Model file for the job. Use its own axes, mm. Face numbers are marked on the shaded views. Coordinates: 2 decimals unless noted, no trailing zeros. Write each loop counter-clockwise with the first axis right and the second up, starting at its lowest first coordinate (ties: lowest second). Pieces come first, ordered by that corner, then holes. Notation, with made-up numbers: M 19,-25.5 L 44,-25.5 A24 cw 44,-0.5 Z; hole C 41,-18.75 d5. An arc over 180 degrees is marked long. Use CSV: the item, a comma, the result in double quotes. Start each with the question number.
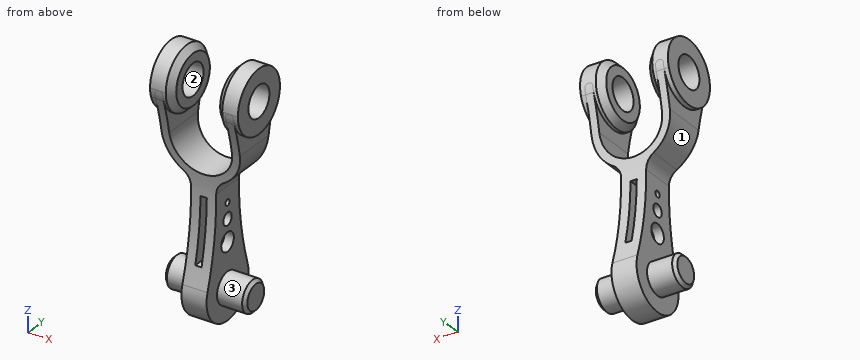
from build123d import *

# Parameters (mm, degrees)
F1_DEPTH  = 19.05
F3_R      = 12.7
F4_DEPTH  = 17.78
F2_R      = 6.35
F6_DEPTH  = 38.1
F5_W      = 17.78
F5_H      = 38.1
F7_DEPTH  = 19.05
F8_SIZE   = 2.54
F10_DEPTH = 5.08
F11_R     = 6.35
F12_DEPTH = 16.51
F13_SIZE  = 1.27
F15_DEPTH = 38.1
F16_W     = 2.54
F16_H     = 25.4
F17_DEPTH = 25.4
F18_R     = 3.81
F18_R_2   = 2.54
F18_R_3   = 1.27
F19_DEPTH = 12.7
F20_ANGLE = 179.9946913403


with BuildPart() as f1:
    # F0 (on Front) → F1 (new body, symmetric)
    with BuildSketch(Plane.XZ):
        with BuildLine():
            ThreePointArc((-5.08, -13.9496366999), (-5.9049678847, -17.0795760164), (-8.1655181496, -19.3962556739))
            ThreePointArc((-8.1655181496, -19.3962556739), (-13.8198807904, -25.1910159629), (-15.8833905736, -33.02))
            Line((-15.8833905736, -33.02), (-15.8833905736, -49.276))
            ThreePointArc((-15.8833905736, -49.276), (-15.4370213081, -50.3536307345), (-14.3593905736, -50.8))
            Line((-14.3593905736, -50.8), (-14.224, -50.8))
            ThreePointArc((-14.224, -50.8), (-13.1463692655, -50.3536307345), (-12.7, -49.276))
            Line((-12.7, -49.276), (-12.7, -33.02))
            ThreePointArc((-12.7, -33.02), (0, -20.32), (12.7, -33.02))
            Line((12.7, -33.02), (12.7, -49.276))
            ThreePointArc((12.7, -49.276), (13.1463692655, -50.3536307345), (14.224, -50.8))
            Line((14.224, -50.8), (14.3593905736, -50.8))
            ThreePointArc((14.3593905736, -50.8), (15.4370213081, -50.3536307345), (15.8833905736, -49.276))
            Line((15.8833905736, -49.276), (15.8833905736, -33.02))
            ThreePointArc((15.8833905736, -33.02), (13.8198807904, -25.1910159629), (8.1655181496, -19.3962556739))
            ThreePointArc((8.1655181496, -19.3962556739), (5.9049678847, -17.0795760164), (5.08, -13.9496366999))
            Line((5.08, -13.9496366999), (5.08, 2.3491094791))
            Line((5.08, 2.3491094791), (-5.08, 2.3491094791))
            Line((-5.08, 2.3491094791), (-5.08, -13.9496366999))
        make_face()
    extrude(amount=F1_DEPTH, both=True)

    # F3 (on Right) → F4 (join, symmetric)
    with BuildSketch(Plane.YZ):
        with Locations((0, -50.8)):
            Circle(F3_R)
    extrude(amount=F4_DEPTH, both=True)

    # F2 (on Right) → F6 (cut, symmetric)
    with BuildSketch(Plane.YZ):
        with Locations((0, -50.8)):
            Circle(F2_R)
    extrude(amount=F6_DEPTH, both=True, mode=Mode.SUBTRACT)

    # F5 (on Front) → F7 (cut, symmetric)
    with BuildSketch(Plane.XZ):
        with Locations((0, -50.8)):
            Rectangle(F5_W, F5_H)
    extrude(amount=F7_DEPTH, both=True, mode=Mode.SUBTRACT)

    # F8
    f8_edges = [f1.edges().sort_by_distance(p)[0] for p in [
        (-8.89, -12.7, -50.8),
        (8.89, -12.7, -50.8),
    ]]
    chamfer(f8_edges, length=F8_SIZE)

    # F9 (on Right) → F10 (join, symmetric)
    with BuildSketch(Plane.YZ):
        with BuildLine():
            Line((19.0499954742, -0.0131314098), (19.0499954742, 25.3868685902))
            ThreePointArc((19.0499954742, 25.3868685902), (0, 44.45), (-19.0499954742, 25.3868685902))
            Line((-19.0499954742, 25.3868685902), (-19.0499954742, -0.0131314098))
            Line((-19.0499954742, -0.0131314098), (19.0499954742, -0.0131314098))
        make_face()
    extrude(amount=F10_DEPTH, both=True)

    # F11 (on Right) → F12 (join, symmetric)
    with BuildSketch(Plane.YZ):
        with Locations((0, 25.4)):
            Circle(F11_R)
    extrude(amount=F12_DEPTH, both=True)

    # F13
    f13_edges = [f1.edges().sort_by_distance(p)[0] for p in [
        (-16.51, -6.35, 25.4),
        (16.51, -6.35, 25.4),
    ]]
    chamfer(f13_edges, length=F13_SIZE)

    # F14 (on Right) → F15 (intersect, symmetric)
    with BuildSketch(Plane.YZ):
        with BuildLine():
            ThreePointArc((12.115027858, -46.99), (6.85027858, -12.7), (12.115027858, 21.59))
            ThreePointArc((12.115027858, 21.59), (0, 38.1), (-12.115027858, 21.59))
            ThreePointArc((-12.115027858, 21.59), (-6.85027858, -12.7), (-12.115027858, -46.99))
            ThreePointArc((-12.115027858, -46.99), (0, -63.5), (12.115027858, -46.99))
        make_face()
    extrude(amount=F15_DEPTH, both=True, mode=Mode.INTERSECT)

    # F16 (on Front) → F17 (cut, symmetric)
    with BuildSketch(Plane.XZ):
        with Locations((0, 1.2903633001)):
            Rectangle(F16_W, F16_H)
    extrude(amount=F17_DEPTH, both=True, mode=Mode.SUBTRACT)

    # F18 (on Right) → F19 (cut, symmetric)
    with BuildSketch(Plane.YZ):
        with Locations((0, 7.62)):
            Circle(F18_R)
        with Locations((0, -1.27)):
            Circle(F18_R_2)
        with Locations((0, -7.62)):
            Circle(F18_R_3)
    extrude(amount=F19_DEPTH, both=True, mode=Mode.SUBTRACT)


with BuildPart() as f1_1:
    # F20: moved
    add(f1.part.rotate(Axis((15.24, 0, 25.4), (1, 0, 0)), F20_ANGLE))


with BuildPart() as f1_2:
    # F22: moved
    add(f1_1.part.moved(Location((0, 0, -101.5999996729))))


solid = f1_2.part
1) Band-saw the part on C-C on z = -66. List the corners of the cut face in (x, y).
2) Band-saw the part on B-B on y = 0. State how many separate pieces and enclosed holes the cut face has, then the cut area to 3 significant figures.
3) Wall check: L1, parallel to X at y = 4.25, z = -48; L2, parallel to Z at x = 5, y = 2; L3, parallel to X at y = -1, z = -18. Give the ranges that are in metal, low to high. Write a range as [from, to].
4) Band-saw the part on A-A on x = -10. List the corners of the cut face in (y, z), then the cut area to 3 significant figures.
5) Two-plate mould, pull along Y, no slides. Class the marked faces 1, 2 and 3: pulls with the +Y half, pulls with the -Y half, needs draft (parallel to the pull), parting line crosses it, or undercut.
6) Drop flat-ended pins along their axis: P1, Ø3, axis at x = 10.5, z = -72.5, coming from the -Y side; P2, Ø8, axis at y = -2, z = -75.5, coming from the +X side; P3, Ø8, axis at y = -2.5, z = -76, coming from the -X side; P4, Ø3, axis at y = 0, z = -49.53, coming from the +X side. Give the stop position or say it passes through.
Findings below:
1,outline,"M -5.08,-10.31 L 5.08,-10.31 L 5.08,10.31 L -5.08,10.31 Z"
2,separate pieces,"8"
2,enclosed holes,"0"
2,area,"1,060 mm2"
3,L1,"x = [-5.08, -1.27], [1.27, 5.08]"
3,L2,"z = [-88.74, -61.66], [-55.18, -51.1], [-47.96, -29.45]"
3,L3,"x = [-15.88, -12.7], [12.7, 15.88]"
4,outline,"C 0.01,0 d22.54; M -7.53,-25.61 A114.3 cw -7.12,-30.12 L 7.13,-30.12 A114.3 cw 7.54,-25.61 Z; C 0,-76.2 d12.7; hole C 0.01,0 d12.7"
4,area,"465 mm2"
5,face 1,"needs draft"
5,face 2,"undercut"
5,face 3,"parting line crosses it"
6,P1,"stops at y = -5.96"
6,P2,"stops at x = 16.51"
6,P3,"stops at x = -16.51"
6,P4,"passes through"
